Can you work these out from the model? Positions are in its coordinate system, mm. Give positions to 0.01 mm unless a question says otherwise; leave off trailing zeros. Write each loop counter-clockwise with the first axis right and the second up, starting at its lowest first coordinate (ties: lowest second). Pieces come first, ordered by that corner, then holes. Notation, with made-up numbers: M -15,53 L -7,53 A20 cw -7,66 Z; hole C 70.25,-7 d4. An arc over 180 degrees is marked long. Use CSV: the item, a comma, the result in double quotes. Start each with the question number.
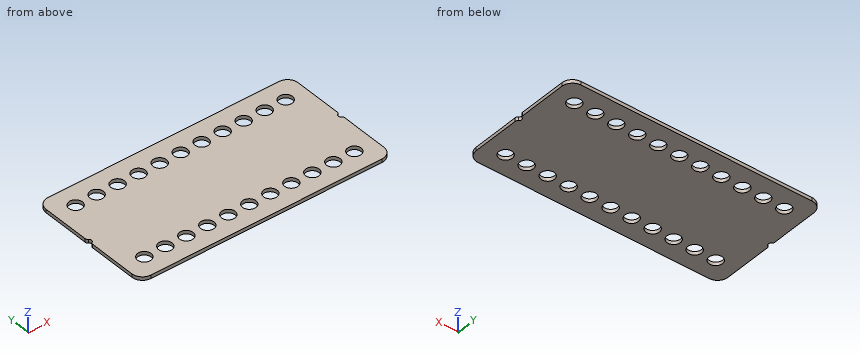
from build123d import *

# Parameters (mm, degrees)
F0_R     = 4.064
F1_DEPTH = 2.1082


with BuildPart() as f1:
    # F0 (on Top) → F1 (new body)
    with BuildSketch(Plane.XY):
        with BuildLine():
            Line((69.85, 38.1), (-69.85, 38.1))
            ThreePointArc((-69.85, 38.1), (-74.340128, 36.240128), (-76.2, 31.75))
            Line((-76.2, 31.75), (-76.2, 2.749631))
            ThreePointArc((-76.2, 2.749631), (-75.987315, 1.955881), (-75.40625, 1.374815))
            ThreePointArc((-75.40625, 1.374815), (-74.6125, 0), (-75.40625, -1.374815))
            ThreePointArc((-75.40625, -1.374815), (-75.987315, -1.955881), (-76.2, -2.749631))
            Line((-76.2, -2.749631), (-76.2, -31.75))
            ThreePointArc((-76.2, -31.75), (-74.340128, -36.240128), (-69.85, -38.1))
            Line((-69.85, -38.1), (69.85, -38.1))
            ThreePointArc((69.85, -38.1), (74.340128, -36.240128), (76.2, -31.75))
            Line((76.2, -31.75), (76.2, -2.749631))
            ThreePointArc((76.2, -2.749631), (75.987315, -1.955881), (75.40625, -1.374815))
            ThreePointArc((75.40625, -1.374815), (74.6125, 0), (75.40625, 1.374815))
            ThreePointArc((75.40625, 1.374815), (75.987315, 1.955881), (76.2, 2.749631))
            Line((76.2, 2.749631), (76.2, 31.75))
            ThreePointArc((76.2, 31.75), (74.340128, 36.240128), (69.85, 38.1))
        make_face()
        with Locations((-63.5, -25.4)):
            Circle(F0_R, mode=Mode.SUBTRACT)
        with Locations((-50.8, -25.4)):
            Circle(F0_R, mode=Mode.SUBTRACT)
        with Locations((-38.1, -25.4)):
            Circle(F0_R, mode=Mode.SUBTRACT)
        with Locations((-25.4, -25.4)):
            Circle(F0_R, mode=Mode.SUBTRACT)
        with Locations((-12.7, -25.4)):
            Circle(F0_R, mode=Mode.SUBTRACT)
        with Locations((0, -25.4)):
            Circle(F0_R, mode=Mode.SUBTRACT)
        with Locations((12.7, -25.4)):
            Circle(F0_R, mode=Mode.SUBTRACT)
        with Locations((25.4, -25.4)):
            Circle(F0_R, mode=Mode.SUBTRACT)
        with Locations((38.1, -25.4)):
            Circle(F0_R, mode=Mode.SUBTRACT)
        with Locations((50.8, -25.4)):
            Circle(F0_R, mode=Mode.SUBTRACT)
        with Locations((63.5, -25.4)):
            Circle(F0_R, mode=Mode.SUBTRACT)
        with Locations((-63.5, 25.4)):
            Circle(F0_R, mode=Mode.SUBTRACT)
        with Locations((-50.8, 25.4)):
            Circle(F0_R, mode=Mode.SUBTRACT)
        with Locations((-38.1, 25.4)):
            Circle(F0_R, mode=Mode.SUBTRACT)
        with Locations((-25.4, 25.4)):
            Circle(F0_R, mode=Mode.SUBTRACT)
        with Locations((-12.7, 25.4)):
            Circle(F0_R, mode=Mode.SUBTRACT)
        with Locations((0, 25.4)):
            Circle(F0_R, mode=Mode.SUBTRACT)
        with Locations((12.7, 25.4)):
            Circle(F0_R, mode=Mode.SUBTRACT)
        with Locations((25.4, 25.4)):
            Circle(F0_R, mode=Mode.SUBTRACT)
        with Locations((38.1, 25.4)):
            Circle(F0_R, mode=Mode.SUBTRACT)
        with Locations((50.8, 25.4)):
            Circle(F0_R, mode=Mode.SUBTRACT)
        with Locations((63.5, 25.4)):
            Circle(F0_R, mode=Mode.SUBTRACT)
    extrude(amount=-F1_DEPTH)


solid = f1.part
(1) Please list where these lines run through material, in increasing order: L1, parallel to Y at x = 0, z = -0.5; L2, parallel to Y at x = -62.5, z = -0.5; L3, parallel to X at y = 32, z = -0.45. Write a range as [from, to].
(2) I want a section at B-B (z = -1.6). State how many separate pieces and enclosed holes the cut face has, and give its area (3 significant figures).
(3) I want a section at A-A (x = 25.4). Write out the boundary of the cut face in (y, z).
(4) Will this pin go through, and if not, where does the flat tip stop? pin 1 Ø13 at (x, y) = (0, 25.4) entering from +Z.
Geometry results:
1,L1,"y = [-38.1, -29.46], [-21.34, 21.34], [29.46, 38.1]"
1,L2,"y = [-38.1, -29.34], [-21.46, 21.46], [29.34, 38.1]"
1,L3,"x = [-76.2, 76.2]"
2,separate pieces,"1"
2,enclosed holes,"22"
2,area,"10,400 mm2"
3,outline,"M -38.1,-2.11 L -29.46,-2.11 L -29.46,0 L -38.1,0 Z; M -21.34,-2.11 L 21.34,-2.11 L 21.34,0 L -21.34,0 Z; M 29.46,-2.11 L 38.1,-2.11 L 38.1,0 L 29.46,0 Z"
4,pin 1,"stops at z = 0"
